Design review of the part built by this model. Coordinates are the model's own, in mm. A direction names the side the tool comes from. Give positions to 0.01 mm unless a question says otherwise; leave off trailing zeros. Loops run counter-clockwise (first coordinate to the right, second up) from the corner with the lowest first, then second, coordinate; pieces in that order, holes last. Notation, with made-up numbers: (-23, -40) - (6, -40) arc R15 ccw to (6, -36) - close; hole circle Ø7 at (49, -27.75). An arc over 180 degrees is marked (long way). Write each question's results on one line, items separated by ' | '.
Autodesk Inventor part; units mm, degrees
ref_plane "YZ Plane" through (0, 0, 0) normal (1, 0, 0) x (0, 1, 0)
ref_plane "XZ Plane" through (0, 0, 0) normal (0, 1, 0) x (-1, 0, 0)
ref_plane "XY Plane" through (0, 0, 0) normal (0, 0, 1) x (1, 0, 0)
sketch "Sketch1" plane through (0, 0, 0) normal (0, 0, 1) x (1, 0, 0)
  circle A0 centre (0, 0) radius 2.032
  circle A1 centre (0, 25.4) radius 2.1082
  line L0 (26.0246, 26.6073) -> (26.0246, 1.2073)
  line L1 (21.8082, 26.6073) -> (21.8082, 1.2073)
  arc A2 (26.0246, 26.6073) -> (21.8082, 26.6073) centre (23.9164, 26.6073) ccw
  arc A3 (21.8082, 1.2073) -> (26.0246, 1.2073) centre (23.9164, 1.2073) ccw
  line L2 (-33.02, 2.1806) -> (-33.02, 33.0568)
  line L3 (33.02, 2.1806) -> (33.02, 33.0568)
  line L4 (0, 43.18) -> (0.8943, 43.18)
  line L5 (0, 43.18) -> (-0.8943, 43.18)
  line L6 (1.6353, 43.0923) -> (30.586, 36.1442)
  line L7 (-1.6353, 43.0923) -> (-30.586, 36.1442)
  line L8 (0, 0) -> (0, -12.7)
  line L9 (-30.9848, -0.7828) -> (-1.1398, -12.2616)
  line L10 (30.9848, -0.7828) -> (1.1398, -12.2616)
  arc A4 (-30.586, 36.1442) -> (-33.02, 33.0568) centre (-29.845, 33.0568) ccw
  arc A5 (-0.8943, 43.18) -> (-1.6353, 43.0923) centre (-0.8943, 40.005) ccw
  arc A6 (1.6353, 43.0923) -> (0.8943, 43.18) centre (0.8943, 40.005) ccw
  arc A7 (33.02, 33.0568) -> (30.586, 36.1442) centre (29.845, 33.0568) ccw
  arc A8 (30.9848, -0.7828) -> (33.02, 2.1806) centre (29.845, 2.1806) ccw
  arc A9 (-1.1398, -12.2616) -> (1.1398, -12.2616) centre (0, -9.2983) ccw
  arc A10 (-33.02, 2.1806) -> (-30.9848, -0.7828) centre (-29.845, 2.1806) ccw
  line L11 (-24.7754, 26.6073) -> (-24.7754, 1.2073)
  line L12 (-28.9918, 26.6073) -> (-28.9918, 1.2073)
  arc A11 (-24.7754, 26.6073) -> (-28.9918, 26.6073) centre (-26.8836, 26.6073) ccw
  arc A12 (-28.9918, 1.2073) -> (-24.7754, 1.2073) centre (-26.8836, 1.2073) ccw
  circle A13 centre (-29.845, 33.0568) radius 2.1082
  circle A14 centre (29.845, 33.0568) radius 2.1082
  point P0 (0, 0)
  point P1 (-33.02, 0)
  point P2 (33.02, 0)
  point P3 (-33.02, 35.56)
  point P4 (1.27, 43.18)
  point P5 (-1.27, 43.18)
  dimension "d1" = 4.2164
  dimension "d10" = 33.02
  dimension "d11" = 33.02
  dimension "d12" = 43.18
  dimension "d13" = 35.56
  dimension "d14" = 1.27
  dimension "d15" = 1.27
  dimension "d16" = 12.7
  dimension "d17" = 3.175
  dimension "d37" = 2.1082
  dimension "d38" = 25.4
  dimension "d39" = 4.2164
  dimension "d41" = 2.1082
  dimension "d43" = 4.2164
  dimension "d44" = 4.2164
  dimension "d45" = 4.2164
extrude "Extrusion3" add sketch "Sketch1" along normal blind 1.524
equation "\"d1\" = d43"
equation "\"d39\" = 2 * d37"
equation "\"d41\" = d37"
equation "\"d43\" = d39"
Item 1: Draft analysis for pull direction X (two halves, no side actions). For faces 1 (the face through (26.025, 14, 1)), 2 (the face through (33.02, 17, 1)), 3 (the face through (-15.908, 39.667, 0.751)), state which applies: +X half, -X half, draft (parallel to the pull), parting line (faces both ways), or undercut.
Output values:
face 1: undercut | face 2: +X half | face 3: -X half
Item 2: We need section C-C on y = 24. Give the boundary of the cut face in (x, z), then the cut area to 3 significant figures.
Output values:
outline: (-33.02, 0) - (-28.99, 0) - (-28.99, 1.52) - (-33.02, 1.52) - close; (-24.78, 0) - (-1.58, 0) - (-1.58, 1.52) - (-24.78, 1.52) - close; (1.58, 0) - (21.81, 0) - (21.81, 1.52) - (1.58, 1.52) - close; (26.02, 0) - (33.02, 0) - (33.02, 1.52) - (26.02, 1.52) - close | area: 83.0 mm²
Item 3: We need section D-D on y = 0. Give the boundary of the cut face in (x, z).
Output values:
outline: (-32.15, 0) - (-28.61, 0) - (-28.61, 1.52) - (-32.15, 1.52) - close; (-25.16, 0) - (-2.03, 0) - (-2.03, 1.52) - (-25.16, 1.52) - close; (2.03, 0) - (22.19, 0) - (22.19, 1.52) - (2.03, 1.52) - close; (25.64, 0) - (32.15, 0) - (32.15, 1.52) - (25.64, 1.52) - close
Item 4: We need section A-A on x = 0. Give the boundary of the cut face in (y, z), then the cut area to 3 significant figures.
Output values:
outline: (-12.47, 0) - (-2.03, 0) - (-2.03, 1.52) - (-12.47, 1.52) - close; (2.03, 0) - (23.29, 0) - (23.29, 1.52) - (2.03, 1.52) - close; (27.51, 0) - (43.18, 0) - (43.18, 1.52) - (27.51, 1.52) - close | area: 72.2 mm²
Item 5: We need section B-B on z = 0.9. Give the boundary of the cut face in (x, y) (1 decimal), then the cut area to 3 significant figures.
Output values:
outline: (-33, 2.2) arc R3.2 ccw to (-31, -0.8) - (-1.1, -12.3) arc R3.2 ccw to (1.1, -12.3) - (31, -0.8) arc R3.2 ccw to (33, 2.2) - (33, 33.1) arc R3.2 ccw to (30.6, 36.1) - (1.6, 43.1) arc R3.2 ccw to (0.9, 43.2) - (-0.9, 43.2) arc R3.2 ccw to (-1.6, 43.1) - (-30.6, 36.1) arc R3.2 ccw to (-33, 33.1) - close; hole circle Ø4.2 at (-29.8, 33.1); hole (-29, 1.2) arc R2.1 ccw to (-24.8, 1.2) - (-24.8, 26.6) arc R2.1 ccw to (-29, 26.6) - close; hole circle Ø4.2 at (0, 25.4); hole circle Ø4.1 at (0, 0); hole (21.8, 1.2) arc R2.1 ccw to (26, 1.2) - (26, 26.6) arc R2.1 ccw to (21.8, 26.6) - close; hole circle Ø4.2 at (29.8, 33.1) | area: 2,730 mm²
Item 6: Clearance check with flat-ended pins moving along their axes: P1, Ø5.5, axis at x = 29.84, y = 33.06, coming from the -Z side; P2, Ø4, axis at x = 0, y = 25.4, coming from the -Z side. State where each tip first meets the part, or that it passes through.
Output values:
P1: stops at z = 0 | P2: passes through
Item 7: Wall thickness on probe 1 along X at (y, z) = (22, 0.8); probe 2 along X at (y, z) = (26, 0.1); probe 3 along X at (y, z) = (31.5, 0.45): over which ranges is each line inside the solid? List them lowest first.
Output values:
probe 1: x = -33.02 to -28.99, -24.78 to 21.81, 26.02 to 33.02 | probe 2: x = -33.02 to -28.99, -24.78 to -2.02, 2.02 to 21.81, 26.02 to 33.02 | probe 3: x = -33.02 to -31.27, -28.42 to 28.42, 31.27 to 33.02
Item 8: Tool access review of faces 4 (the face through (0, 16, 0)), 5 (the face through (24, -0.9, 0.8)): name each direction out of +Z, -Z, +X, -X, +Y, -Y from which nothing blocks a thin tool from reaching the whole face with its end or side.
Output values:
face 4: -Z, +X, -X, +Y, -Y | face 5: +Z, -Z
